from build123d import *

# Parameters (mm, degrees)
F0_W     = 101.6
F0_H     = 101.6
F0_W_2   = 88.9
F0_H_2   = 88.9
F1_DEPTH = 609.6
F2_R     = 5.08
F3_R     = 12.7
F4_DEPTH = 101.601


with BuildPart() as f1:
    # F0 (on Front) → F1 (new body, symmetric)
    with BuildSketch(Plane.XZ):
        Rectangle(F0_W, F0_H)
        Rectangle(F0_W_2, F0_H_2, mode=Mode.SUBTRACT)
    extrude(amount=F1_DEPTH, both=True)

    # F2
    f2_edges = [f1.edges().sort_by_distance(p)[0] for p in [
        (-50.8, 0, 50.8),
        (50.8, 0, 50.8),
        (50.8, 0, -50.8),
        (-50.8, 0, -50.8),
    ]]
    fillet(f2_edges, radius=F2_R)

    # F3 (on face) → F4 (cut, through all)
    with BuildSketch(Plane.XY.offset(50.8)):
        with Locations((0, 523.160219)):
            Circle(F3_R)
        with Locations((0, 446.960219)):
            Circle(F3_R)
        with Locations((0, 370.760219)):
            Circle(F3_R)
        with Locations((0, 294.560219)):
            Circle(F3_R)
        with Locations((0, 218.360219)):
            Circle(F3_R)
        with Locations((0, 142.160219)):
            Circle(F3_R)
        with Locations((0, 65.960219)):
            Circle(F3_R)
        with Locations((0, -10.239781)):
            Circle(F3_R)
        with Locations((0, -86.439781)):
            Circle(F3_R)
        with Locations((0, -162.639781)):
            Circle(F3_R)
    extrude(amount=-F4_DEPTH, mode=Mode.SUBTRACT)


solid = f1.part
Design review of the part built by this model. Coordinates are the model's own, in mm. A direction names the side the tool comes from. Give positions to 0.01 mm unless a question says otherwise; leave off trailing zeros. Loops run counter-clockwise (first coordinate to the right, second up) from the corner with the lowest first, then second, coordinate; pieces in that order, holes last. Notation, with made-up numbers: M 17,48.25 L 53,48.25 A12 ccw 53,53.25 Z; hole C 75.5,60 d8. An arc over 180 degrees is marked long. Write item = value, one per line.
Q1. Draft analysis for pull direction X (two halves, no side actions). For faces 1 (the cylindrical face through (-2.75, -22.64, 47.67)), 2 (the cylindrical face through (-1.653, 383.352, 47.669)), 3 (the flat face through (50.8, -9, -1)), 4 (the flat face through (20, -9, 50.8)), state which applies: +X half, -X half, draft (parallel to the pull), parting line (faces both ways), or undercut.
Output values:
face_1 = undercut
face_2 = undercut
face_3 = +X half
face_4 = draft
Q2. We need section C-C (y = 471.5). Give the boundary of the cut face in (x, z).
Output values:
outline = M -50.8,-45.72 A5.08 ccw -45.72,-50.8 L 45.72,-50.8 A5.08 ccw 50.8,-45.72 L 50.8,45.72 A5.08 ccw 45.72,50.8 L -45.72,50.8 A5.08 ccw -50.8,45.72 Z; hole M -44.45,-44.45 L 44.45,-44.45 L 44.45,44.45 L -44.45,44.45 Z
Q3. We need section B-B (x = 26.5). Give the boundary of the cut face in (y, z), plus the area to 3 significant figures.
Output values:
outline = M -609.6,-50.8 L 609.6,-50.8 L 609.6,-44.45 L -609.6,-44.45 Z; M -609.6,44.45 L 609.6,44.45 L 609.6,50.8 L -609.6,50.8 Z
area = 15,500 mm^2
Q4. We need section A-A (z = 3). Give the boundary of the cut face in (x, y).
Output values:
outline = M -50.8,-609.6 L -44.45,-609.6 L -44.45,609.6 L -50.8,609.6 Z; M 44.45,-609.6 L 50.8,-609.6 L 50.8,609.6 L 44.45,609.6 Z
Q5. To check wall thickness, follow line 1 (Z direction, x = 40, y = 213.5). State the ranges of the line that lie inside material, in increasing order. Write a range as [from, to].
Output values:
line_1 = [-50.8, -44.45], [44.45, 50.8]
Q6. Insertion check: pin 1 (23 mm diameter, centred on x = 0, y = 218.36, fed in from +Z). The pin has a flat end and moves straight along its axis. Give the tip position at first contact, or say it passes through.
Output values:
pin_1 = through
Q7. For faces 5 (the flat face through (19, -9, -44.45)), 6 (the flat face through (-45, -609.6, 0)), list the 3-axis set-ups (+Z, -Z, +X, -X, +Y, -Y) from which the entire face can be reached by the end or side of a thin tool; tool diameter is ignored.
Output values:
face_5 = +Y, -Y
face_6 = +Z, -Z, +X, -X, -Y
